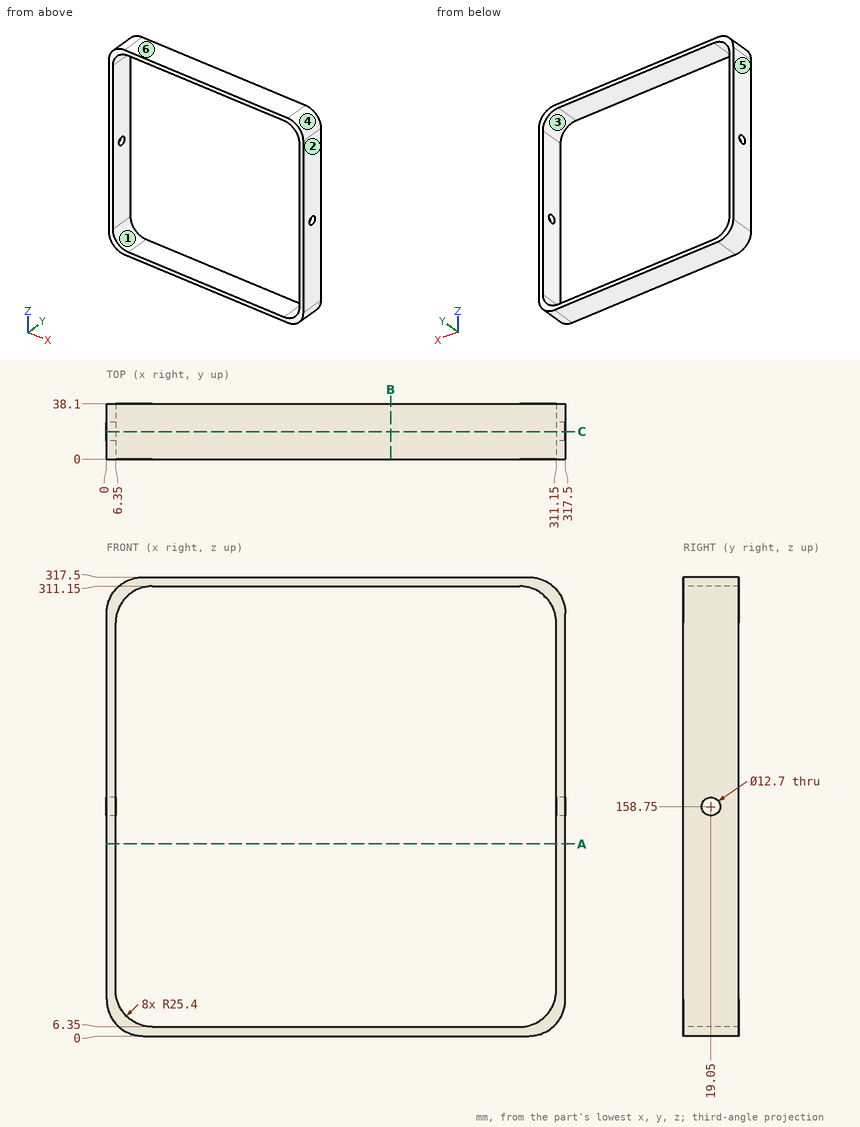
For this review, use the dimensioned drawing (mm, ordinates from the lowest corner) and the shaded views. A direction names the side the tool comes from. Give positions to 0.01 mm unless a question says otherwise; leave off trailing zeros. Loops run counter-clockwise (first coordinate to the right, second up) from the corner with the lowest first, then second, coordinate; pieces in that order, holes last.
Item 1: Take a section at B-B, the plane x = 196.5. State the section outline as (y, z) points, and give its area (3 significant figures).
Item 2: For line 1 along X through (y, z) = (15.5, 63.5); line 2 along X through (y, z) = (11, 13), list the stretches that pass through material, from the lowest coordinate up.
Item 3: Tool access review of the marked faces 1 and 2: name each direction out of +Z, -Z, +X, -X, +Y, -Y from which nothing blocks a thin tool from reaching the whole face with its end or side.
Item 4: Take a section at C-C, the plane y = 19.05. State the section outline as (x, z) points, and give its area (3 significant figures).
Item 5: Draft analysis for pull direction X (two halves, no side actions). For the marked faces 3, 4, 5 and 6, state which applies: +X half, -X half, draft (parallel to the pull), parting line (faces both ways), or undercut.
Item 6: Take a section at A-A, the plane z = 133. State the section outline as (x, y) points.
Calculated:
1. outline: (0, 0) - (38.1, 0) - (38.1, 6.35) - (0, 6.35) - close; (0, 311.15) - (38.1, 311.15) - (38.1, 317.5) - (0, 317.5) - close
1. area: 484 mm2
2. line 1: x = 0 to 6.35, 311.15 to 317.5
2. line 2: x = 3.23 to 14.62, 302.88 to 314.27
3. face 1: +Y, -Y
3. face 2: +Z, -Z, +X, +Y, -Y
4. outline: (0, 25.4) arc R25.4 ccw to (25.4, 0) - (292.1, 0) arc R25.4 ccw to (317.5, 25.4) - (317.5, 152.4) - (311.15, 152.4) - (311.15, 31.75) arc R25.4 cw to (285.75, 6.35) - (31.75, 6.35) arc R25.4 cw to (6.35, 31.75) - (6.35, 152.4) - (0, 152.4) - close; (0, 165.1) - (6.35, 165.1) - (6.35, 285.75) arc R25.4 cw to (31.75, 311.15) - (285.75, 311.15) arc R25.4 cw to (311.15, 285.75) - (311.15, 165.1) - (317.5, 165.1) - (317.5, 292.1) arc R25.4 ccw to (292.1, 317.5) - (25.4, 317.5) arc R25.4 ccw to (0, 292.1) - close
4. area: 7,740 mm2
5. face 3: undercut
5. face 4: +X half
5. face 5: -X half
5. face 6: draft
6. outline: (0, 0) - (6.35, 0) - (6.35, 38.1) - (0, 38.1) - close; (311.15, 0) - (317.5, 0) - (317.5, 38.1) - (311.15, 38.1) - close
